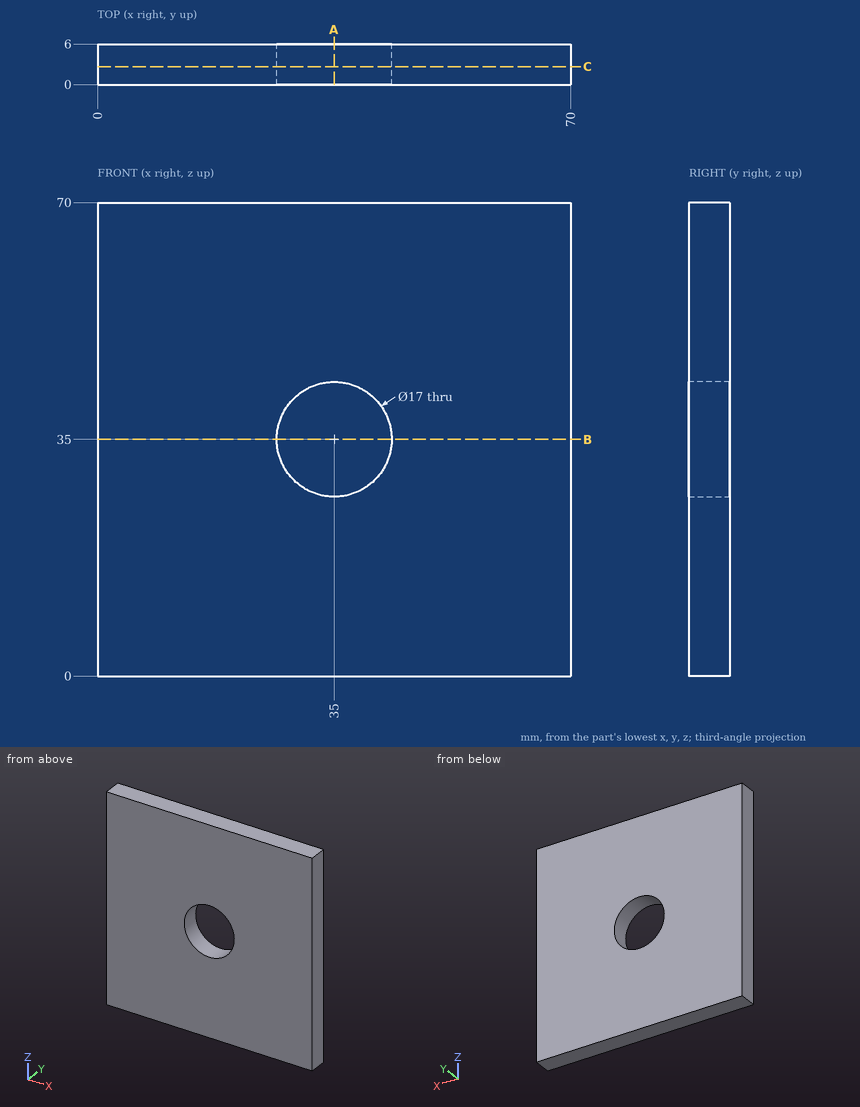
Here's the drawing with two shaded views (mm, measured from the low corner). I have some questions. Round coordinates to 2 decimals unless told otherwise and drop trailing zeros. Loops run counter-clockwise (first coordinate to the right, second up) from the corner with the lowest first, then second, coordinate; pieces in that order, holes last. Notation, with made-up numbers: (86, -3.75) -> (124, -3.75) arc R16 cw to (124, 18.25) -> close; hole circle Ø6 at (-29.5, 77.5). An arc over 180 degrees is marked (long way). Answer as CSV lines item,"result". Start each with the question number.
1. Imagine slicing it at C-C on y = 2.65. Write out the boundary of the cut face in (x, z).
2. I need wall thicknesses on probe 1 along X at (y, z) = (1.8, 35.5); probe 2 along X at (y, z) = (3, 36). Which ranges of each line are inside material? Lowest first, please. Write a range as from..to.
3. Imagine slicing it at A-A on x = 35. Write out the boundary of the cut face in (y, z).
4. Imagine slicing it at B-B on z = 35. Write out the boundary of the cut face in (x, y), plus the area to 3 significant figures.
Solution:
1,outline,"(0, 0) -> (70, 0) -> (70, 70) -> (0, 70) -> close; hole circle Ø17 at (35, 35)"
2,probe 1,"0..26.51, 43.49..70"
2,probe 2,"0..26.56, 43.44..70"
3,outline,"(0, 0) -> (6, 0) -> (6, 26.5) -> (0, 26.5) -> close; (0, 43.5) -> (6, 43.5) -> (6, 70) -> (0, 70) -> close"
4,outline,"(0, 0) -> (26.5, 0) -> (26.5, 6) -> (0, 6) -> close; (43.5, 0) -> (70, 0) -> (70, 6) -> (43.5, 6) -> close"
4,area,"318 mm²"
